The figure shows three views and two pictorial views of one solid part (mm, origin at its lowest corner). Answer the questions. Round coordinates to 2 decimals unless told otherwise and drop trailing zeros. Write each loop counter-clockwise with the first axis right and the second up, starting at its lowest first coordinate (ties: lowest second). Pieces come first, ordered by that corner, then holes. Notation, with made-up numbers: M 65,-2.5 L 116,-2.5 A31 ccw 116,21.5 Z; hole C 43,80.25 d7. An arc over 180 degrees is marked long. One line per item, written item: value. Start each with the question number.
Q1. Given pin 1 Ø8 at (x, y) = (11, 3.5) entering from -Z; pin 2 Ø3.5 at (x, y) = (11, 11) entering from +Z; pin 3 Ø2 at (x, z) = (10, 7.5) entering from -Y; pin 4 Ø2 at (y, z) = (9.5, 10) entering from -X, each flat-ended and moving along its own axis, determine where each tip first touches the part or whether it passes through.
Q2. Find section A-A (x = 8). Write down the section's boundary in (y, z), and give its area (3 significant figures).
Q3. The mould has two halves that part along Y. Classify the marked faces 1, 2 and 3: released by +Y, released by -Y, zero draft, split by the parting line, or undercut.
Q4. Find section B-B (z = 9.25). Write down the section's boundary in (x, y), and give its area (3 significant figures).
Q5. Consider probe 1 along Y at (x, z) = (8, 7); probe 2 along Z at (x, y) = (8, 2.5); probe 3 along Y at (x, z) = (13.5, 10.25). Determine where each line is inside the solid, lowest interval first.
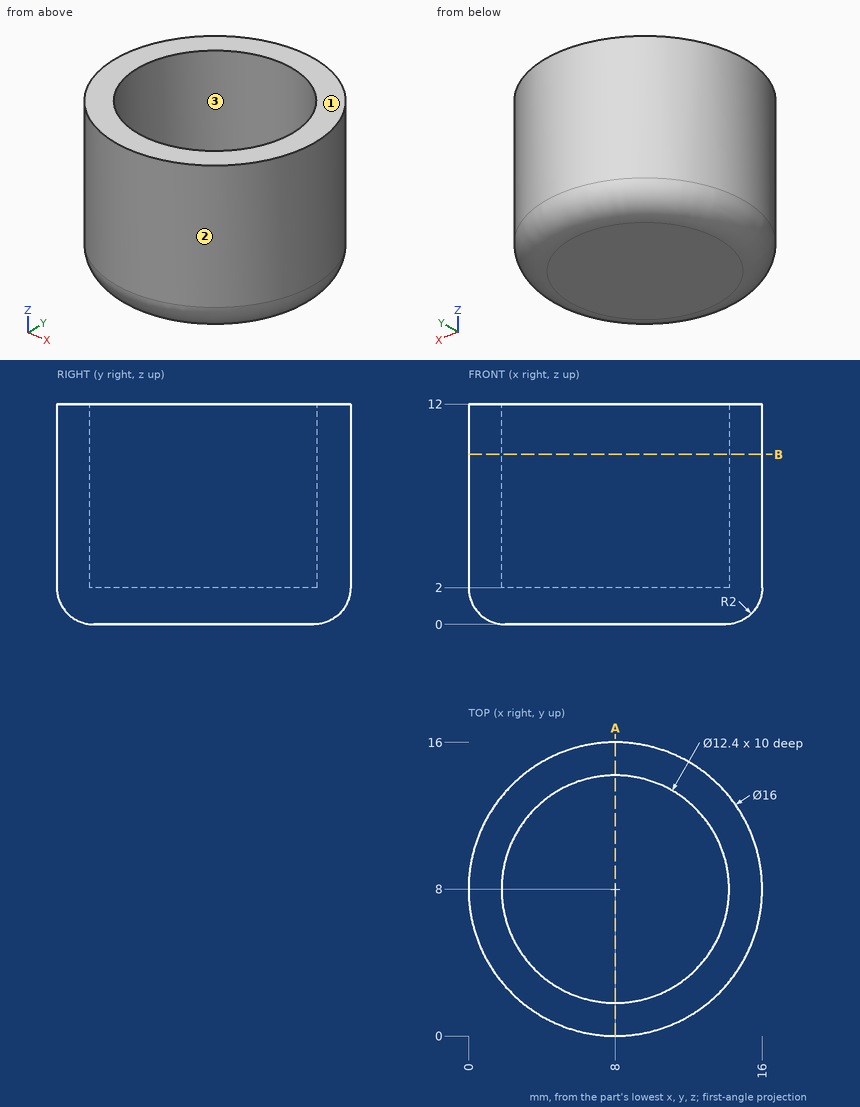
The answers:
1. pin 1: z = 0
1. pin 2: z = 2
1. pin 3: y = 0.06
1. pin 4: x = 0.02
2. outline: M 0,2 A2 ccw 2,0 L 14,0 A2 ccw 16,2 L 16,12 L 14.2,12 L 14.2,2 L 1.8,2 L 1.8,12 L 0,12 Z
2. area: 66.3 mm2
3. face 1: zero draft
3. face 2: split by the parting line
3. face 3: undercut
4. outline: C 8,8 d16; hole C 8,8 d12.4
4. area: 80.3 mm2
5. probe 1: 0 to 1.8, 14.2 to 16
5. probe 2: 0 to 2
5. probe 3: 2.19 to 5.14, 10.86 to 13.81
